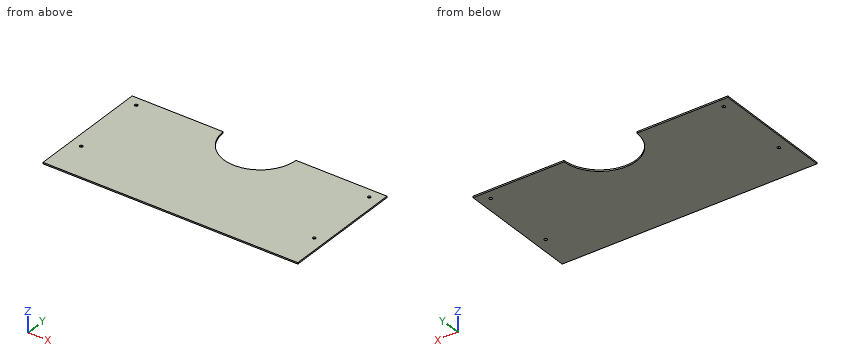
Autodesk Inventor part; units mm, degrees
ref_plane "YZ Plane" through (0, 0, 0) normal (1, 0, 0) x (0, 1, 0)
ref_plane "XZ Plane" through (0, 0, 0) normal (0, 1, 0) x (-1, 0, 0)
ref_plane "XY Plane" through (0, 0, 0) normal (0, 0, 1) x (1, 0, 0)
sketch "Sketch1" plane through (0, 0, 0) normal (0, 0, 1) x (1, 0, 0)
  line L0 (0, 0) -> (542, 0)
  line L1 (542, 0) -> (542, 261)
  line L2 (0, 261) -> (0, 0)
  line L3 (271, 0) -> (271, 263)
  arc A0 (193.5258, 261) -> (348.4742, 261) centre (271, 263) ccw
  line L4 (542, 261) -> (348.4742, 261)
  line L5 (193.5258, 261) -> (0, 261)
  dimension "d0" = 542
  dimension "d24" = 155
  dimension "d25" = 263
  dimension "d26" = 261
extrude "Extrusion1" add sketch "Sketch1" along normal blind 3
sketch "Sketch2" plane through (0, 0, 0) normal (0, 0, -1) x (-1, 0, 0)
  line L0 (0, 261) -> (0, 0)
  line L1 (-542, 0) -> (-542, 261)
  line L2 (-542, 261) -> (0, 261)
  point P0 (-23, 241)
  point P1 (-23, 80)
  point P2 (-519, 241)
  point P3 (-519, 80)
  dimension "d4" = 23
  dimension "d13" = 20
  dimension "d14" = 261
  dimension "d15" = 542
  dimension "d18" = 161
  dimension "d21" = 496
hole "Hole1" at (23, 241, 0) at (519, 241, 0) at (519, 80, 0) at (23, 80, 0) direction (0, 0, 1) diameter 6.5 end through all
properties part number "plate_top_03" material "Polystyrene"
Here's how the part is built. I have some questions about the finished solid (model axes, mm). Round coordinates to 2 decimals unless told otherwise and drop trailing zeros. Loops run counter-clockwise (first coordinate to the right, second up) from the corner with the lowest first, then second, coordinate; pieces in that order, holes last. Notation, with made-up numbers: (-2, -38.75) - (13, -38.75) arc R11 cw to (13, -29.75) - close; hole circle Ø8 at (44, 40.5). An arc over 180 degrees is marked (long way). One line per question, with ' | ' between items. Start each with the question number.
Q1. I want a section at C-C (x = 271). Write out the boundary of the cut face in (y, z).
Q2. I want a section at A-A (z = 1). Write out the boundary of the cut face in (x, y).
Q3. I want a section at B-B (y = 191). Write out the boundary of the cut face in (x, z).
Q4. Please list where these lines run through material, in increasing order: line 1 (Y direction, x = 23, z = 1.8); line 2 (X direction, y = 80, z = 0.8); line 3 (X direction, y = 241, z = 1.6). Write a range as [from, to].
Response values:
1) outline: (0, 0) - (185.5, 0) - (185.5, 3) - (0, 3) - close
2) outline: (0, 0) - (542, 0) - (542, 261) - (348.47, 261) arc R77.5 cw to (193.53, 261) - (0, 261) - close; hole circle Ø6.5 at (23, 80); hole circle Ø6.5 at (23, 241); hole circle Ø6.5 at (519, 80); hole circle Ø6.5 at (519, 241)
3) outline: (0, 0) - (242.33, 0) - (242.33, 3) - (0, 3) - close; (299.67, 0) - (542, 0) - (542, 3) - (299.67, 3) - close
4) line 1: y = [0, 76.75], [83.25, 237.75], [244.25, 261] | line 2: x = [0, 19.75], [26.25, 515.75], [522.25, 542] | line 3: x = [0, 19.75], [26.25, 196.69], [345.31, 515.75], [522.25, 542]
